Drawing for the job (mm, zero at the part's lowest x, y, z). A direction names the side the tool comes from. Round coordinates to 2 decimals unless told otherwise and drop trailing zeros. Write each loop counter-clockwise with the first axis right and the second up, starting at its lowest first coordinate (ties: lowest second). Pieces come first, ordered by that corner, then holes.
Item 1: Band-saw the part on C-C, the plane x = 42. Write the cut outline in (y, z), then the cut area to 3 significant figures.
Item 2: Band-saw the part on D-D, the plane x = 13. Write the cut outline in (y, z) (1 decimal).
Item 3: 3-axis set-ups, long thin cutter, end or side, ignore diameter. For the marked faces 1 and 2: which of +Z, -Z, +X, -X, +Y, -Y reach the whole face in a straight line?
Item 4: Wall check: probe 1 along Y at (x, z) = (20, 8.75); probe 2 along Z at (x, y) = (38, 25.5); probe 3 along Y at (x, z) = (17.5, 2.25). Give the ranges that are in metal, low to high.
Item 5: Band-saw the part on B-B, the plane y = 16. Write the cut outline in (x, z) (1 decimal).
Item 6: Mould opens along Y. For the marked faces 3, 4, 5 and 6 say: +Y half, -Y half, draft (parallel to the pull), parting line (faces both ways), or undercut.
Item 7: Drop flat-ended pins along their axis: pin 1 Ø6 at (x, z) = (51, 16) entering from -Y; pin 2 Ø11 at (x, z) = (44, 15) entering from +Y; pin 3 Ø10 at (x, z) = (53.5, 11.5) entering from +Y; pin 4 Ø3 at (x, z) = (25, 24.5) entering from +Y. Give the stop position or say it passes through.
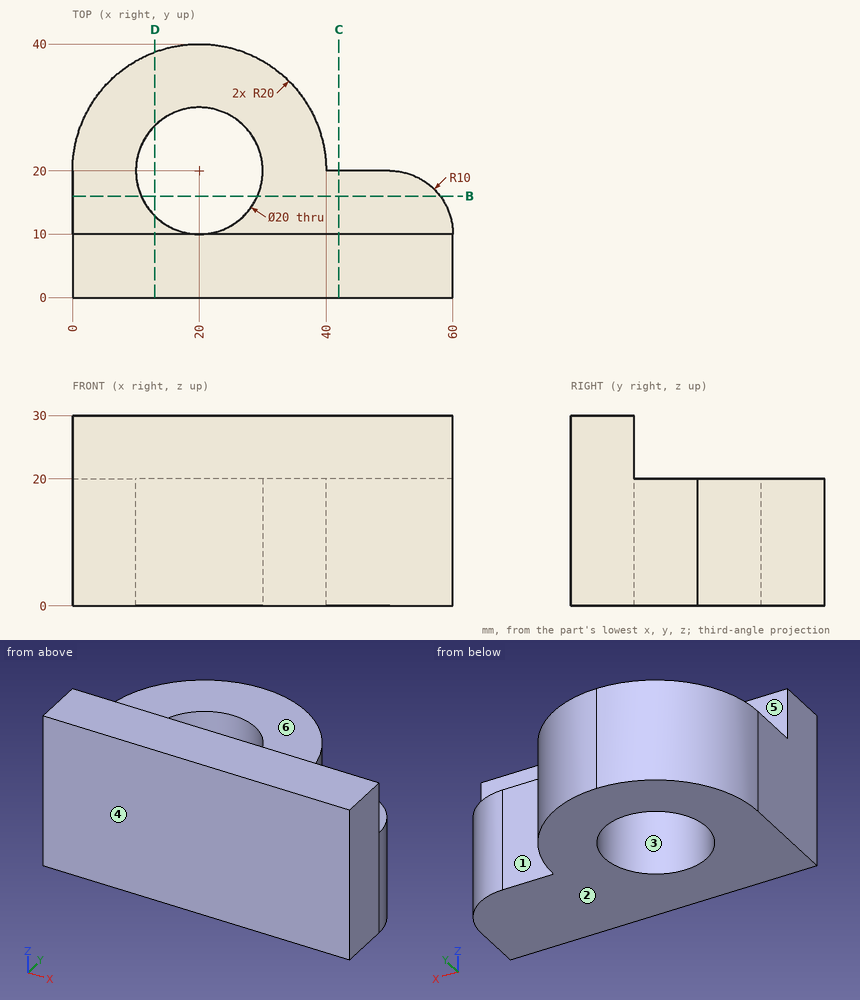
Results:
1. outline: (0, 0) - (20, 0) - (20, 20) - (10, 20) - (10, 30) - (0, 30) - close
1. area: 500 mm2
2. outline: (0, 0) - (12.9, 0) - (12.9, 20) - (10, 20) - (10, 30) - (0, 30) - close; (27.1, 0) - (38.7, 0) - (38.7, 20) - (27.1, 20) - close
3. face 1: +Z, -Z, +X, +Y
3. face 2: -Z, +X, -X, +Y, -Y
4. probe 1: y = 0 to 10, 30 to 40
4. probe 2: z = 0 to 20
4. probe 3: y = 0 to 10.32, 29.68 to 39.84
5. outline: (0, 0) - (10.8, 0) - (10.8, 20) - (0, 20) - close; (29.2, 0) - (58, 0) - (58, 20) - (29.2, 20) - close
6. face 3: undercut
6. face 4: -Y half
6. face 5: +Y half
6. face 6: draft
7. pin 1: stops at y = 0
7. pin 2: stops at y = 27.6
7. pin 3: stops at y = 20
7. pin 4: stops at y = 10
